For this review, take the finished solid that the model builds, in its own axes (mm). A direction names the side the tool comes from. Give positions to 0.01 mm unless a question says otherwise; leave off trailing zeros. Order: outer loops, then holes, each group sorted by start corner. A loop starts at its lowest first (then second) coordinate and runs counter-clockwise, first axis right, second up. Notation, with made-up numbers: M 47.25,-15.5 L 92.25,-15.5 A15 cw 92.25,-11.5 Z; hole C 31,31.5 d5. An arc over 180 degrees is marked long. Use CSV: the item, a comma, the result in double quotes. Start each with the question number.
(1) Tool access review of faces 1 (the face through (-9.764, 199.3, 74.362)), 2 (the face through (507.75, 74, 4)): name each direction out of +Z, -Z, +X, -X, +Y, -Y from which nothing blocks a thin tool from reaching the whole face with its end or side.
(2) Clearance check with flat-ended pins moving along their axes: P1, Ø1.5, axis at x = -233, z = -89.5, coming from the +Y side; P2, Ø1, axis at y = 205, z = -20, coming from the +X side. State where each tip first meets the part, or that it passes through.
(3) Consider section D-D (x = -959). Write out the cut boundary in (y, z).
(4) Consider section B-B (x = 0). Write out the cut boundary in (y, z).
(5) Wall thickness on L1, parallel to Y at x = 143, z = 253; L2, parallel to X at y = 158.5, z = 32: over which ranges is each line inside the solid? List them lowest first. Write a range as from..to.
(6) Consider section A-A (z = 0). Write out the cut boundary in (x, y), and give its area (3 significant figures).
(7) Consider section C-C (y = 226). Write out the cut boundary in (x, z).
Autodesk Inventor part; units mm, degrees
ref_plane "YZ Plane" through (0, 0, 0) normal (1, 0, 0) x (0, 1, 0)
ref_plane "XZ Plane" through (0, 0, 0) normal (0, 1, 0) x (-1, 0, 0)
ref_plane "XY Plane" through (0, 0, 0) normal (0, 0, 1) x (1, 0, 0)
sketch "Sketch1" plane through (0, 0, 0) normal (1, 0, 0) x (0, 1, 0)
  line L0 (0, -300) -> (150, -300)
  line L1 (150, -300) -> (150, 300)
  line L2 (150, 300) -> (0, 300)
  line L3 (0, 300) -> (0, -300)
  line L4 (150, -110.5085) -> (250, -110.5085)
  line L5 (250, -110.5085) -> (250, 120.1522)
  line L6 (250, 120.1522) -> (150, 120.1522)
  line L7 (150, 120.1522) -> (150, -110.5085)
  line L8 (250, -527.4169) -> (326.5108, -527.4169)
  line L9 (326.5108, -527.4169) -> (326.5108, 687.4915)
  line L10 (326.5108, 687.4915) -> (250, 687.4915)
  line L11 (250, 687.4915) -> (250, -527.4169)
  line L12 (326.5108, -527.4169) -> (729.0925, -527.4169)
  line L13 (326.5108, 687.4915) -> (739.1213, 687.4915)
  point P0 (0, 0)
  point P1 (0, 0)
  dimension "d0" = 600
  dimension "d1" = 150
  dimension "d2" = 100
sketch "Sketch2" plane through (0, 0, 0) normal (1, 0, 0) x (0, 1, 0)
  line L0 (0, -300) -> (150, -300)
  line L1 (150, -300) -> (150, 300)
  line L2 (150, 300) -> (0, 300)
  line L3 (0, 300) -> (0, -300)
  point P0 (0, 0)
  point P1 (0, 0)
  dimension "d3" = 600
  dimension "d4" = 150
extrude "Extrusion1" add sketch "Sketch2" along normal blind 507.75 and the other way blind 1159.5
sketch "Sketch3" plane through (-1159.5, 150, 300) normal (0, 1, 0) x (1, 0, 0)
  circle A0 centre (1159.5, 300) radius 75
  dimension "d9" = 150
extrude "Extrusion2" add sketch "Sketch3" along normal blind 100
sketch3d "3D Sketch1"
equation "\"d3\" = d0"
equation "\"d4\" = d1"
equation "\"d10\" = d2"
properties part number "MSC DIM 012 carriage nose"
Check result:
1,face 1,"+Y"
1,face 2,"+Z, -Z, +X, +Y, -Y"
2,P1,"stops at y = 150"
2,P2,"stops at x = 72.42"
3,outline,"M 0,-300 L 150,-300 L 150,300 L 0,300 Z"
4,outline,"M 0,-300 L 150,-300 L 150,-75 L 250,-75 L 250,75 L 150,75 L 150,300 L 0,300 Z"
5,L1,"y = 0..150"
5,L2,"x = -67.83..67.83"
6,outline,"M -1159.5,0 L 507.75,0 L 507.75,150 L 75,150 L 75,250 L -75,250 L -75,150 L -1159.5,150 Z"
6,area,"265,000 mm^2"
7,outline,"C 0,0 d150"
